Input: part model. Units: mm. Frame: model coordinates. A direction names the side the tool comes from. Coordinates: 2 decimals unless noted, no trailing zeros. Order: outer loops, then holes, each group sorted by start corner. A loop starts at its lowest first (then second) coordinate and runs counter-clockwise, first axis right, second up. Notation, with made-up numbers: M 1,-25 L 48,-25 A15 cw 48,-17 Z; hole C -19,24 d2. An arc over 180 degrees is marked long. One line per item, written item: value.
```python
from build123d import *

# Parameters (mm, degrees)
F2_R     = 6
F3_DEPTH = 88.001


with BuildPart() as f1:
    # F0 (on Top) → F1 (revolve)
    with BuildSketch(Plane.XY):
        Polygon((0, 17.928575), (0, 0), (88, 0), (88, 9.928573), (85, 9.928573), (85, 12.928574), (68, 12.928574), (68, 17.928575), align=None)
    revolve(axis=Axis((44, 0, 0), (1, 0, 0)))

    # F2 (on Right) → F3 (cut, through all)
    with BuildSketch(Plane.YZ):
        Circle(F2_R)
    extrude(amount=F3_DEPTH, mode=Mode.SUBTRACT)


solid = f1.part
```
(1) Cut plane C-C on x = 11.5. Output: boundary loops of the cut face in (y, z).
Data:
outline: C 0,0 d35.86; hole C 0,0 d12
(2) Ray query, line 1 (Z direction, x = 61.5, y = 0); line 2 (X direction, y = 11, z = 0); line 3 (Z direction, x = 5, y = -2). Return the intervals inside material, ascending. Write a range as from..to.
Data:
line 1: z = -17.93..-6, 6..17.93
line 2: x = 0..85
line 3: z = -17.82..-5.66, 5.66..17.82
(3) Cut plane A-A on z = 0. Output: boundary loops of the cut face in (x, y), plus the area to 3 significant figures.
Data:
outline: M 0,-17.93 L 68,-17.93 L 68,-12.93 L 85,-12.93 L 85,-9.93 L 88,-9.93 L 88,-6 L 0,-6 Z; M 0,6 L 88,6 L 88,9.93 L 85,9.93 L 85,12.93 L 68,12.93 L 68,17.93 L 0,17.93 Z
area: 1,880 mm2
(4) Access query for faces 1 (the flat face through (88, 0.1, -6.5)), 2 (the flat face through (68, -9.2, 9.4)). Directions: +Z, -Z, +X, -X, +Y, -Y. A direction counts if a zero-diameter tool reaches every point of the face in a straight line with its end or side. Return the directions, or none.
Data:
face 1: +Z, -Z, +X, +Y, -Y
face 2: +X
(5) Draft query along Z for faces 3 (the cylindrical face through (76.381, -10.26, -7.867)), 4 (the flat face through (0, 8, 0)), 5 (the cylindrical face through (43, -6, 0)). Return one class per face: released by +Z, released by -Z, zero draft, split by the parting line, or undercut.
Data:
face 3: split by the parting line
face 4: zero draft
face 5: undercut
(6) First-contact query: pin 1 (3 mm diameter, centred on x = 66, z = -6, fed in from +Y); pin 2 (8 mm diameter, centred on x = 21, z = 11.5, fed in from +Y); pin 3 (2 mm diameter, centred on x = 45.5, z = -6, fed in from +Y). Flat tips, straight axial feed; report the tip coordinate or a pass-through.
Data:
pin 1: stops at y = 17.35
pin 2: stops at y = 16.28
pin 3: stops at y = 17.22
(7) Cut plane D-D on y = 12. Output: boundary loops of the cut face in (x, z), plus the area to 3 significant figures.
Data:
outline: M 0,-13.32 L 68,-13.32 L 68,-4.81 L 85,-4.81 L 85,4.81 L 68,4.81 L 68,13.32 L 0,13.32 Z
area: 1,980 mm2
